from build123d import *

# Parameters (mm, degrees)
SKETCH27_R          = 4
SKETCH27_R_2        = 2.5
BOSS_EXTRUDE1_DEPTH = 6
SKETCH33_R          = 4.99
CUT_EXTRUDE2_DEPTH  = 3
SKETCH34_W          = 24
SKETCH34_H          = 6
CUT_EXTRUDE3_DEPTH  = 3
SKETCH35_R          = 1.5
CUT_EXTRUDE4_DEPTH  = 3
FILLET1_R           = 3
CUT_EXTRUDE5_REACH  = 5
SKETCH36_R          = 1.5
FILLET3_R           = 2
FILLET4_R           = 10


with BuildPart() as part:
    # Sketch27 → Boss-Extrude1 (new body)
    with BuildSketch(Plane(origin=(0, 0, 0), x_dir=(0, 0, -1), z_dir=(1, 0, 0))):
        with BuildLine():
            Line((9, 50), (66, 50))
            Line((66, 50), (66, 45))
            Line((66, 45), (48.564398788, 34))
            Line((48.564398788, 34), (9, 34))
            ThreePointArc((9, 34), (1, 42), (9, 50))
        make_face()
        with Locations((9, 42)):
            Circle(SKETCH27_R, mode=Mode.SUBTRACT)
        with Locations((50, 42)):
            Circle(SKETCH27_R_2, mode=Mode.SUBTRACT)
    extrude(amount=BOSS_EXTRUDE1_DEPTH)

    # Sketch33 → Cut-Extrude2 (cut)
    with BuildSketch(Plane(origin=(6, 0, 0), x_dir=(0, 0, -1), z_dir=(1, 0, 0))):
        with Locations((9, 42)):
            Circle(SKETCH33_R)
    extrude(amount=-CUT_EXTRUDE2_DEPTH, mode=Mode.SUBTRACT)

    # Sketch34 → Cut-Extrude3 (cut)
    with BuildSketch(Plane(origin=(6, 0, 0), x_dir=(0, 0, -1), z_dir=(1, 0, 0))):
        with Locations((32, 37)):
            Rectangle(SKETCH34_W, SKETCH34_H)
    extrude(amount=-CUT_EXTRUDE3_DEPTH, mode=Mode.SUBTRACT)

    # Sketch35 → Cut-Extrude4 (cut)
    with BuildSketch(Plane(origin=(6, 0, 0), x_dir=(0, 0, -1), z_dir=(1, 0, 0))):
        with Locations((21, 39)):
            Circle(SKETCH35_R)
        with Locations((43, 39)):
            Circle(SKETCH35_R)
    extrude(amount=-CUT_EXTRUDE4_DEPTH, mode=Mode.SUBTRACT)

    # Fillet1
    fillet1_edges = [part.edges().sort_by_distance(p)[0] for p in [
        (4.5, 37.881966011, -20),
        (4.5, 40, -22.118033989),
        (4.5, 40, -41.881966011),
        (4.5, 37.881966011, -44),
    ]]
    fillet(fillet1_edges, radius=FILLET1_R)

    # Sketch36 → Cut-Extrude5 (cut, up to next)
    with BuildSketch(Plane(origin=(3, 0, 0), x_dir=(0, 0, -1), z_dir=(1, 0, 0)), mode=Mode.PRIVATE) as cut_extrude5_sk1:
        with Locations((23, 37)):
            Circle(SKETCH36_R)
    cut_extrude5_tool1 = extrude(cut_extrude5_sk1.sketch, amount=-CUT_EXTRUDE5_REACH, mode=Mode.PRIVATE) & part.part
    add(cut_extrude5_tool1.solids().sort_by_distance((3, 37, -23))[0], mode=Mode.SUBTRACT)
    # Sketch36 → Cut-Extrude5 (cut, up to next)
    with BuildSketch(Plane(origin=(3, 0, 0), x_dir=(0, 0, -1), z_dir=(1, 0, 0)), mode=Mode.PRIVATE) as cut_extrude5_sk2:
        with Locations((41, 37)):
            Circle(SKETCH36_R)
    cut_extrude5_tool2 = extrude(cut_extrude5_sk2.sketch, amount=-CUT_EXTRUDE5_REACH, mode=Mode.PRIVATE) & part.part
    add(cut_extrude5_tool2.solids().sort_by_distance((3, 37, -41))[0], mode=Mode.SUBTRACT)

    # Fillet3
    fillet3_edges = [part.edges().sort_by_distance(p)[0] for p in [
        (3, 50, -66),
        (3, 45, -66),
    ]]
    fillet(fillet3_edges, radius=FILLET3_R)

    # Fillet4
    fillet4_edges = [part.edges().sort_by_distance(p)[0] for p in [
        (3, 34, -48.564398788),
    ]]
    fillet(fillet4_edges, radius=FILLET4_R)


solid = part.part
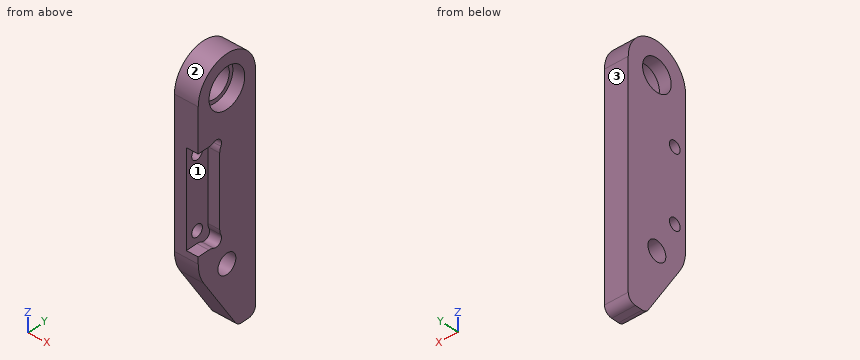
Design review of the part built by this model. Coordinates are the model's own, in mm. Face numbers are marked on the shaded views. Round coordinates to 2 decimals unless told otherwise and drop trailing zeros. Write each loop counter-clockwise with the first axis right and the second up, starting at its lowest first coordinate (ties: lowest second). Pieces come first, ordered by that corner, then holes. Notation, with made-up numbers: (-38.5, 85.5) - (-18.5, 85.5) arc R21 cw to (-18.5, 89.5) - close; hole circle Ø6 at (67, 17). An arc over 180 degrees is marked (long way). Use a Markdown table: item, result. Add a question column.
1. Mouldability with a two-part tool opening along Z and no side actions: class the marked faces 1, 2 and 3 as +Z half, -Z half, draft (parallel to the pull), parting line (faces both ways), or undercut.
2. Wall thickness on probe 1 along Y at (x, z) = (0.9, -41); probe 2 along Y at (x, z) = (4.75, -9); probe 3 along Z at (x, y) = (0.6, 43.5): over which ranges is each line inside the solid? List them lowest first.
3. We need section B-B (z = -48.5). State the section outline as (x, y) points, then the cut area to 3 significant figures.
4. We need section A-A (x = 4.1). State the section outline as (y, z) points.
5. Clearance check with flat-ended pins moving along their axes: pin 1 (3 mm diameter, centred on x = 1, y = 42, fed in from -Z); pin 2 (3.5 mm diameter, centred on x = 5, z = -36, fed in from -Y); pin 3 (0.9 mm diameter, centred on x = 4, y = 35.5, fed in from +Z). State where each tip first meets the part, or that it passes through.
6. We need section C-C (y = 42). State the section outline as (x, z) points, then the cut area to 3 significant figures.
7. We need section D-D (z = -27). State the section outline as (x, y) points, then the cut area to 3 significant figures.
Output:
| question | item | result |
|---|---|---|
| 1 | face 1 | undercut |
| 1 | face 2 | +Z half |
| 1 | face 3 | draft |
| 2 | probe 1 | y = 34 to 35.5, 38.5 to 50 |
| 2 | probe 2 | y = 34 to 37.01, 46.99 to 50 |
| 2 | probe 3 | z = -63.62 to -52, -48 to -12.71, -5.29 to -1.14 |
| 3 | outline | (0, 34.41) - (6, 34.41) - (6, 40) - (0, 40) - close; (0, 44) - (6, 44) - (6, 50) - (0, 50) - close |
| 3 | area | 69.6 mm2 |
| 4 | outline | (34, -45.67) arc R10 ccw to (35.54, -51.01) - (44.41, -65.07) arc R2 ccw to (46.1, -66) - (48, -66) arc R2 ccw to (50, -64) - (50, -9) arc R8 ccw to (34, -9) - (34, -20) - (36.94, -20) arc R3 ccw to (38.31, -19.67) arc R1.5 cw to (40.33, -21.69) arc R3 ccw to (40, -23.06) - (40, -40.94) arc R3 ccw to (40.33, -42.31) arc R1.5 cw to (38.31, -44.33) arc R3 ccw to (36.94, -44) - (34, -44) - close; hole circle Ø9.98 at (42, -9); hole circle Ø5 at (42, -50) |
| 5 | pin 1 | stops at z = -63.62 |
| 5 | pin 2 | stops at y = 40 |
| 5 | pin 3 | stops at z = -3.77 |
| 6 | outline | (0, -61.24) - (6, -61.24) - (6, -52.5) - (0, -52.5) - close; (0, -47.5) - (6, -47.5) - (6, -13.99) - (3, -13.99) - (3, -13) - (0, -13) - close; (0, -5) - (3, -5) - (3, -4.01) - (6, -4.01) - (6, -1) - (0, -1) - close |
| 6 | area | 278 mm2 |
| 7 | outline | (0, 34) - (3, 34) - (3, 40) - (6, 40) - (6, 50) - (0, 50) - close |
| 7 | area | 78.0 mm2 |
